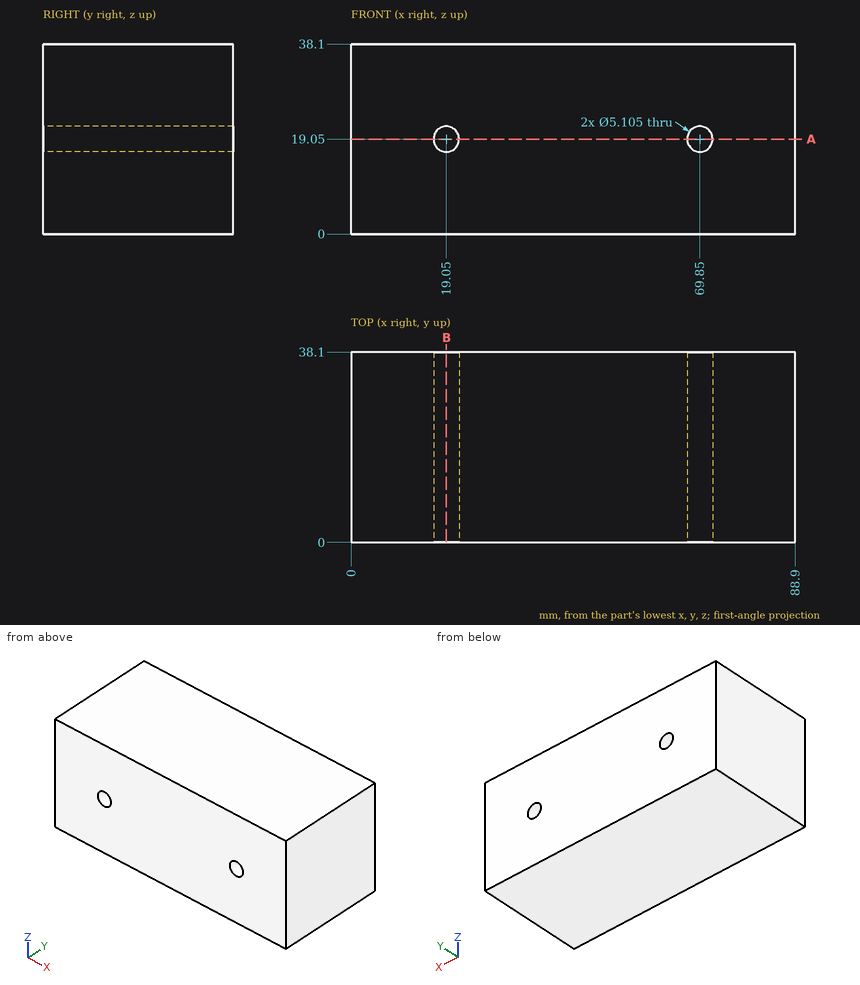
Answer from the drawing. Dimensions are ordinates in mm from the lowest x, y and z of the part. Give positions to 0.01 mm unless a question says otherwise; leave off trailing zeros. Write each loop counter-clockwise with the first axis right and the second up, starting at its lowest first coordinate (ties: lowest second). Pieces come first, ordered by that corner, then holes.
1) Section A-A (z = 19.05) is taken. Write down the section's boundary in (x, y), and give its area (3 significant figures).
2) Section B-B (x = 19.05) is taken. Write down the section's boundary in (y, z), and give its area (3 significant figures).
3) Find the intervals of material crossed by L1, parallel to X at y = 10, z = 19; L2, parallel to Z at x = 69.85, y = 22; L3, parallel to X at y = 9.5, z = 17.5, in increasing order.
Response:
1. outline: (0, 0) - (16.5, 0) - (16.5, 38.1) - (0, 38.1) - close; (21.6, 0) - (67.3, 0) - (67.3, 38.1) - (21.6, 38.1) - close; (72.4, 0) - (88.9, 0) - (88.9, 38.1) - (72.4, 38.1) - close
1. area: 3,000 mm2
2. outline: (0, 0) - (38.1, 0) - (38.1, 16.5) - (0, 16.5) - close; (0, 21.6) - (38.1, 21.6) - (38.1, 38.1) - (0, 38.1) - close
2. area: 1,260 mm2
3. L1: x = 0 to 16.5, 21.6 to 67.3, 72.4 to 88.9
3. L2: z = 0 to 16.5, 21.6 to 38.1
3. L3: x = 0 to 17.02, 21.08 to 67.82, 71.88 to 88.9
